Verification items for this drawing (mm, ordinates from the low corner). Give positions to 0.01 mm unless a question says otherwise; leave off trailing zeros. Loops run counter-clockwise (first coordinate to the right, second up) from the corner with the lowest first, then second, coordinate; pieces in that order, holes last. Notation, with made-up numbers: (4.25, 78) - (24.25, 78) arc R23 ccw to (24.25, 117) - close; hole circle Ø1 at (22, -18). An arc over 180 degrees is marked (long way). One line per question, with ' | ' between items. Start each with the question number.
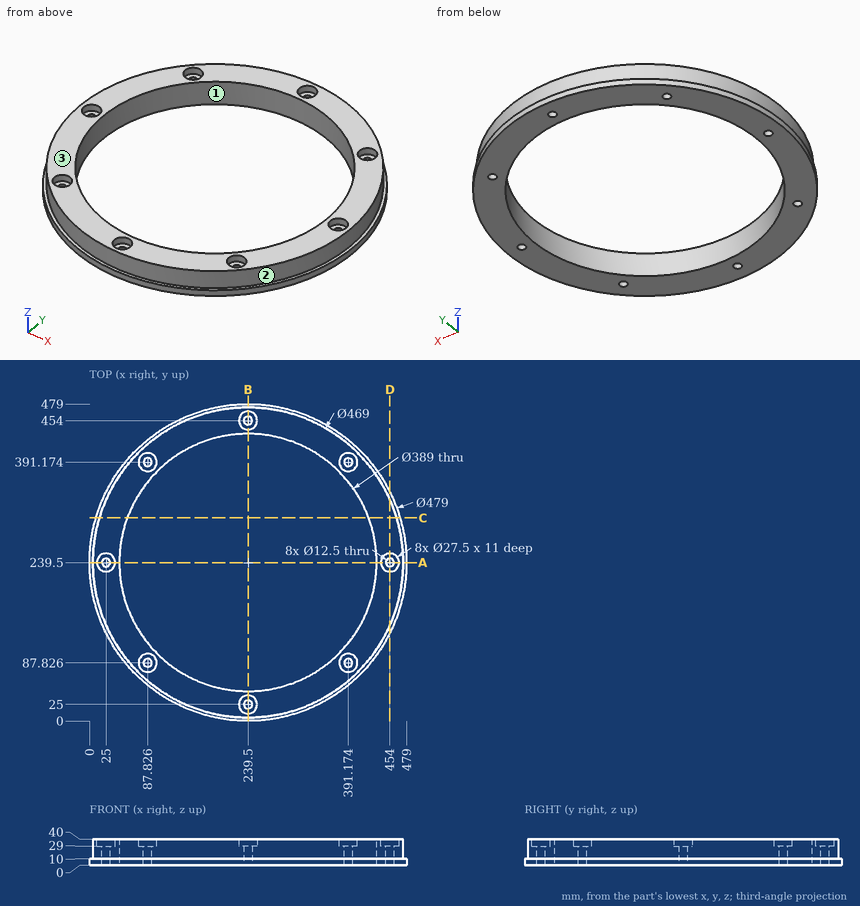
(1) Section check C-C, the plane y = 307. Record the boundary of the cut face in (x, z) (1 decimal), and give its area (3 significant figures).
(2) Material ranges on line 1 (Y direction, x = 239, z = 18); line 2 (X direction, y = 108.5, z = 32.5); line 3 (X direction, y = 345.5, z = 11) (1 decimal), recorded low to high.
(3) Mould release check, pull along Y, two halves, no side actions. Record for the marked faces 1, 2 and 3: pulls with the +Y half, pulls with the -Y half, needs draft (parallel to the pull), parting line crosses it, or undercut.
(4) Section check D-D, the plane x = 454. Record the boundary of the cut face in (y, z).
(5) Section check A-A, the plane y = 239.5. Record the boundary of the cut face in (x, z).
(6) Depth check by flat-ended pin: pin 1 Ø2 at (x, z) = (384.5, 6.5) entering from -Y (1 decimal); pin 2 Ø1 at (x, z) = (282, 30.5) entering from +Y; pin 3 Ø8 at (x, z) = (178, 21) entering from -Y. Enter the tip coordinate at first touch or a pass-through.
Numbers:
1) outline: (9.7, 0) - (57.1, 0) - (57.1, 40) - (14.9, 40) - (14.9, 10) - (9.7, 10) - close; (421.9, 0) - (469.3, 0) - (469.3, 10) - (464.1, 10) - (464.1, 40) - (421.9, 40) - close | area: 3,480 mm^2
2) line 1: 5 to 18.77, 31.23 to 45, 434 to 447.77, 460.23 to 474 | line 2: 45 to 95.73, 383.27 to 434 | line 3: 30.3 to 76.4, 402.6 to 448.7
3) face 1: undercut | face 2: parting line crosses it | face 3: needs draft
4) outline: (132.96, 0) - (233.25, 0) - (233.25, 29) - (225.75, 29) - (225.75, 40) - (144.74, 40) - (144.74, 10) - (132.96, 10) - close; (245.75, 0) - (346.04, 0) - (346.04, 10) - (334.26, 10) - (334.26, 40) - (253.25, 40) - (253.25, 29) - (245.75, 29) - close
5) outline: (0, 0) - (18.75, 0) - (18.75, 29) - (11.25, 29) - (11.25, 40) - (5, 40) - (5, 10) - (0, 10) - close; (31.25, 0) - (45, 0) - (45, 40) - (38.75, 40) - (38.75, 29) - (31.25, 29) - close; (434, 0) - (447.75, 0) - (447.75, 29) - (440.25, 29) - (440.25, 40) - (434, 40) - close; (460.25, 0) - (479, 0) - (479, 10) - (474, 10) - (474, 40) - (467.75, 40) - (467.75, 29) - (460.25, 29) - close
6) pin 1: y = 48.1 | pin 2: y = 470.21 | pin 3: y = 12.16
